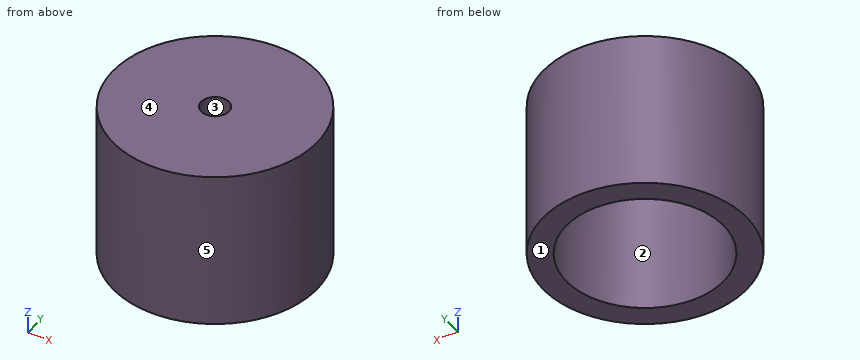
from build123d import *

# Parameters (mm, degrees)
F0_R     = 5.5
F0_R_2   = 4.25
F1_DEPTH = 8.5
F2_DEPTH = 7
F3_D     = 1.5


with BuildPart() as f1:
    # F0 (on Top) → F1 (new body)
    with BuildSketch(Plane.XY):
        with Locations((0, -0.5465864819)):
            Circle(F0_R)
        with Locations((0, -0.5465864819)):
            Circle(F0_R_2, mode=Mode.SUBTRACT)
        with Locations((0, -0.5465864819)):
            Circle(F0_R_2)
    extrude(amount=F1_DEPTH)

    # F0 (on Top) → F2 (cut)
    with BuildSketch(Plane.XY):
        with Locations((0, -0.5465864819)):
            Circle(F0_R_2)
    extrude(amount=F2_DEPTH, mode=Mode.SUBTRACT)

    # F3 (through all)
    with Locations(Plane(origin=(0, 0, 0), x_dir=(1, 0, 0), z_dir=(0, 0, -1))):
        with Locations((0, 0.5465864819)):
            Hole(F3_D / 2)


solid = f1.part
Can you work these out from the model? Positions are in its coordinate system, mm. Face numbers are marked on the shaded views. A direction names the side the tool comes from. Round coordinates to 2 decimals unless told otherwise and drop trailing zeros. Order: outer loops, then holes, each group sorted by start corner. A loop starts at its lowest first (then second) coordinate and runs counter-clockwise, first axis right, second up. Notation, with made-up numbers: (60.5, -40) -> (64.5, -40) arc R13 ccw to (64.5, -29) -> close; hole circle Ø9 at (-9, 3). An arc over 180 degrees is marked (long way). Write each question's results on one line, items separated by ' | '. Start each with the question number.
Item 1: Which directions (+Z, -Z, +X, -X, +Y, -Y) give clear straight access to the entire face, cutting with the end or side of a thin tool? Please do the marked faces 1 and 2.
Item 2: Will these pins go through, and if not, where does the flat tip stop? pin 1 (1.5 mm diameter, centred on y = -3.5, z = 1.5, fed in from -X); pin 2 (5 mm diameter, centred on y = 3.5, z = 1, fed in from -X); pin 3 (4 mm diameter, centred on x = 4, z = 2, fed in from -Y).
Item 3: Thinking about a two-plate mould opening in Y: for the marked faces 3, 4 and 5, which applies, +Y half, -Y half, draft (parallel to the pull), parting line (faces both ways), or undercut?
Item 4: If we section it at C-C, the plane x = -3: Write out the boundary of the cut face in (y, z).
Item 5: If we section it at A-A, the plane x = 0: Write out the boundary of the cut face in (y, z).
Item 6: Please list where these lines run through material, in increasing order: L1, parallel to Y at x = 0, z = 5.5; L2, parallel to Y at x = 0, z = 8.05; L3, parallel to X at y = -0.5, z = 1.
Item 7: If we section it at D-D, the plane z = 1.5: Write out the boundary of the cut face in (x, y), then the cut area to 3 significant figures.
Item 8: If we section it at B-B, the plane y = 0.75: Write out the boundary of the cut face in (x, z), then the cut area to 3 significant figures.
Results:
1) face 1: -Z, +X, -X, +Y, -Y | face 2: -Z
2) pin 1: stops at x = -5.04 | pin 2: stops at x = -5.28 | pin 3: stops at y = -5.67
3) face 3: undercut | face 4: draft | face 5: parting line
4) outline: (-5.16, 0) -> (-3.56, 0) -> (-3.56, 7) -> (2.46, 7) -> (2.46, 0) -> (4.06, 0) -> (4.06, 8.5) -> (-5.16, 8.5) -> close
5) outline: (-6.05, 0) -> (-4.8, 0) -> (-4.8, 7) -> (-1.3, 7) -> (-1.3, 8.5) -> (-6.05, 8.5) -> close; (0.2, 7) -> (3.7, 7) -> (3.7, 0) -> (4.95, 0) -> (4.95, 8.5) -> (0.2, 8.5) -> close
6) L1: y = -6.05 to -4.8, 3.7 to 4.95 | L2: y = -6.05 to -1.3, 0.2 to 4.95 | L3: x = -5.5 to -4.25, 4.25 to 5.5
7) outline: circle Ø11 at (0, -0.55); hole circle Ø8.5 at (0, -0.55) | area: 38.3 mm2
8) outline: (-5.34, 0) -> (-4.05, 0) -> (-4.05, 7) -> (4.05, 7) -> (4.05, 0) -> (5.34, 0) -> (5.34, 8.5) -> (-5.34, 8.5) -> close | area: 34.2 mm2
